```python
from build123d import *

# Parameters (mm, degrees)
F0_W     = 50
F0_H     = 40
F1_DEPTH = 40
F2_W     = 10
F2_H     = 20
F3_DEPTH = 50.001
F4_W     = 30
F4_H     = 10
F5_DEPTH = 20.001
F6_W     = 10
F6_H     = 20
F7_DEPTH = 20
F8_W     = 10
F8_H     = 20
F9_DEPTH = 30.001


with BuildPart() as f1:
    # F0 (on Front) → F1 (new body)
    with BuildSketch(Plane.XZ):
        with Locations((25, 20)):
            Rectangle(F0_W, F0_H)
    extrude(amount=F1_DEPTH)

    # F2 (on face) → F3 (cut, through all)
    with BuildSketch(Plane(origin=(0, 0, 0), x_dir=(0, -1, 0), z_dir=(-1, 0, 0))):
        with Locations((5, 30)):
            Rectangle(F2_W, F2_H)
        with Locations((35, 30)):
            Rectangle(F2_W, F2_H)
    extrude(amount=-F3_DEPTH, mode=Mode.SUBTRACT)

    # F4 (on face) → F5 (cut, through all)
    with BuildSketch(Plane.XY.offset(20)):
        with Locations((15, -5)):
            Rectangle(F4_W, F4_H)
        with Locations((15, -35)):
            Rectangle(F4_W, F4_H)
    extrude(amount=-F5_DEPTH, mode=Mode.SUBTRACT)

    # F6 (on face) → F7 (cut, through all)
    with BuildSketch(Plane.XY.offset(40)):
        with Locations((45, -20)):
            Rectangle(F6_W, F6_H)
    extrude(amount=-F7_DEPTH, mode=Mode.SUBTRACT)

    # F8 (on face) → F9 (cut, through all)
    with BuildSketch(Plane.XZ.offset(30)):
        with Locations((5, 30)):
            Rectangle(F8_W, F8_H)
        Polygon((10, 20), (0, 20), (0, 0), align=None)
    extrude(amount=-F9_DEPTH, mode=Mode.SUBTRACT)


solid = f1.part
```
Verification items for the finished model (mm, model axes). A direction names the side the tool comes from. Give positions to 0.01 mm unless a question says otherwise; leave off trailing zeros. Order: outer loops, then holes, each group sorted by start corner. A loop starts at its lowest first (then second) coordinate and runs counter-clockwise, first axis right, second up. Notation, with made-up numbers: (14, 22) -> (46, 22) arc R20 ccw to (46, 61) -> close; hole circle Ø9 at (-9.75, 25). An arc over 180 degrees is marked (long way). Use a Markdown table: item, result.
1) Material ranges on probe 1 along Y at (x, z) = (6, 6); probe 2 along Z at (x, y) = (46, -29.5); probe 3 along X at (y, z) = (-11.5, 23), recorded low to high.
Results:
| item | result |
|---|---|
| probe 1 | -30 to -10 |
| probe 2 | 0 to 20 |
| probe 3 | 10 to 40 |
2) Section check A-A, the plane x = 34. Record the boundary of the cut face in (y, z).
Results:
| item | result |
|---|---|
| outline | (-40, 0) -> (0, 0) -> (0, 20) -> (-10, 20) -> (-10, 40) -> (-30, 40) -> (-30, 20) -> (-40, 20) -> close |
3) Tool access check on faces 1 (the flat face through (30, -35, 10)), 2 (the flat face through (10, -20, 30)), 3 (the flat face through (30, -5, 10)). Record the directions out of +Z, -Z, +X, -X, +Y, -Y that give a thin tool (end or side, any length) a straight path to the whole face; none if there is none.
Results:
| item | result |
|---|---|
| face 1 | +Z, -Z, -X, -Y |
| face 2 | +Z, -X, +Y, -Y |
| face 3 | +Z, -Z, -X, +Y |
4) Depth check by flat-ended pin: pin 1 Ø3 at (y, z) = (-37, 7.5) entering from -X; pin 2 Ø1.5 at (y, z) = (-20.5, 18.5) entering from -X (3 decimals); pin 3 Ø1 at (x, y) = (41.5, -16) entering from +Z. Enter the tip coordinate at first touch or a pass-through.
Results:
| item | result |
|---|---|
| pin 1 | x = 30 |
| pin 2 | x = 8.875 |
| pin 3 | z = 20 |
5) Section check B-B, the plane z = 3.5. Record the boundary of the cut face in (x, y), then the cut area to 4 significant figures.
Results:
| item | result |
|---|---|
| outline | (1.75, -30) -> (30, -30) -> (30, -40) -> (50, -40) -> (50, 0) -> (30, 0) -> (30, -10) -> (1.75, -10) -> close |
| area | 1,365 mm² |
6) Section check D-D, the plane x = 16. Record the boundary of the cut face in (y, z).
Results:
| item | result |
|---|---|
| outline | (-30, 0) -> (-10, 0) -> (-10, 40) -> (-30, 40) -> close |
7) Section check C-C, the plane y = -18. Record the boundary of the cut face in (x, z).
Results:
| item | result |
|---|---|
| outline | (0, 0) -> (50, 0) -> (50, 20) -> (40, 20) -> (40, 40) -> (10, 40) -> (10, 20) -> close |
